from build123d import *

# Parameters (mm, degrees)
AUFSATZ_LINEAR_AUSTRAGEN1_DEPTH = 105
M5_GEWINDEBOHRUNG1_D            = 4.2
M5_GEWINDEBOHRUNG1_DEPTH        = 14
M5_GEWINDEBOHRUNG1_TIP          = 1.2618073
M5_GEWINDEBOHRUNG2_D            = 4.2
M5_GEWINDEBOHRUNG2_DEPTH        = 14
M5_GEWINDEBOHRUNG2_TIP          = 1.2618073
SKIZZE10_R                      = 2.55
SCHNITT_LINEAR_AUSTRAGEN1_DEPTH = 11
G1_4_GEWINDEBOHRUNG1_D          = 11.8


with BuildPart() as part:
    # Skizze1 → Aufsatz-Linear austragen1 (new body, symmetric)
    with BuildSketch(Plane.XY):
        Polygon((-40, 0), (40, 0), (40, 10), (10, 10), (10, 4), (-10, 4), (-10, 10), (-40, 10), align=None)
    extrude(amount=AUFSATZ_LINEAR_AUSTRAGEN1_DEPTH, both=True)

    # M5 Gewindebohrung1
    with Locations(Plane.XY.offset(105)):
        with Locations((-30, 4), (30, 4)):
            Hole(M5_GEWINDEBOHRUNG1_D / 2, depth=M5_GEWINDEBOHRUNG1_DEPTH)
            with Locations((0, 0, -(M5_GEWINDEBOHRUNG1_DEPTH + M5_GEWINDEBOHRUNG1_TIP / 2))):  # 118° drill point
                Cone(0, M5_GEWINDEBOHRUNG1_D / 2, M5_GEWINDEBOHRUNG1_TIP, mode=Mode.SUBTRACT)

    # M5 Gewindebohrung2
    with Locations(Plane(origin=(0, 0, -105), x_dir=(-1, 0, 0), z_dir=(0, 0, -1))):
        with Locations((-25, 4), (25, 4)):
            Hole(M5_GEWINDEBOHRUNG2_D / 2, depth=M5_GEWINDEBOHRUNG2_DEPTH)
            with Locations((0, 0, -(M5_GEWINDEBOHRUNG2_DEPTH + M5_GEWINDEBOHRUNG2_TIP / 2))):  # 118° drill point
                Cone(0, M5_GEWINDEBOHRUNG2_D / 2, M5_GEWINDEBOHRUNG2_TIP, mode=Mode.SUBTRACT)

    # Skizze10 → Schnitt-Linear austragen1 (cut, through all)
    with BuildSketch(Plane(origin=(0, 10, 0), x_dir=(1, 0, 0), z_dir=(0, 1, 0))):
        with Locations((25, 75)):
            Circle(SKIZZE10_R)
        with Locations((25, 45)):
            Circle(SKIZZE10_R)
        with Locations((25, 15)):
            Circle(SKIZZE10_R)
        with Locations((25, -15)):
            Circle(SKIZZE10_R)
        with Locations((25, -45)):
            Circle(SKIZZE10_R)
        with Locations((25, -75)):
            Circle(SKIZZE10_R)
        with Locations((-25, -75)):
            Circle(SKIZZE10_R)
        with Locations((-25, -45)):
            Circle(SKIZZE10_R)
        with Locations((-25, -15)):
            Circle(SKIZZE10_R)
        with Locations((-25, 15)):
            Circle(SKIZZE10_R)
        with Locations((-25, 45)):
            Circle(SKIZZE10_R)
        with Locations((-25, 75)):
            Circle(SKIZZE10_R)
    extrude(amount=-SCHNITT_LINEAR_AUSTRAGEN1_DEPTH, mode=Mode.SUBTRACT)

    # G1/4 Gewindebohrung1 (through all)
    with Locations(Plane(origin=(0, 4, 0), x_dir=(1, 0, 0), z_dir=(0, 1, 0))):
        with Locations((0, 95), (0, -95)):
            Hole(G1_4_GEWINDEBOHRUNG1_D / 2)


solid = part.part
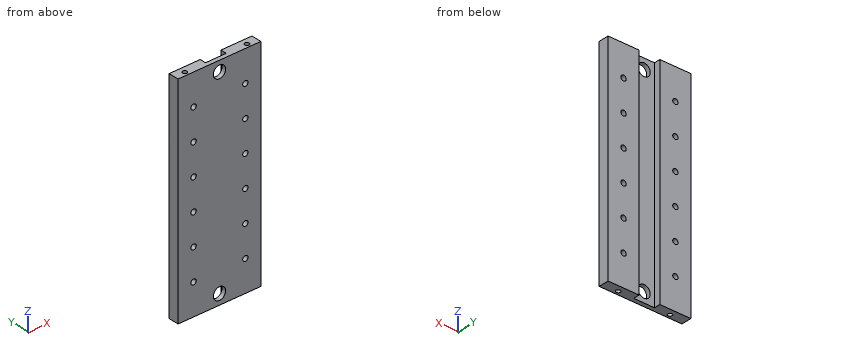
Can you work these out from the model? Positions are in its coordinate system, mm. Round coordinates to 2 decimals unless told otherwise and drop trailing zeros. Order: outer loops, then holes, each group sorted by start corner. A loop starts at its lowest first (then second) coordinate and runs counter-clockwise, first axis right, second up. Notation, with made-up numbers: M -32,87 L -26,87 A12 cw -26,106 Z; hole C -21.75,-10 d1. An arc over 180 degrees is marked long. Use a Markdown table: item, result.
1) I'm going to push flat-ended pins straight in: P1, Ø8, axis at x = -25, z = 15, coming from the +Y side; P2, Ø4, axis at x = 25, y = 4, coming from the -Z side. Where does each tip first touch, or does it pass through?
Geometry says:
| item | result |
|---|---|
| P1 | stops at y = 10 |
| P2 | stops at z = -90.94 |
2) If I drill on line 1 along X through (y, z) = (7.5, -15); line 2 along X through (y, z) = (8, 76.5); line 3 along X through (y, z) = (7.5, 94), over which ranges is the centre line in solid material (lowest first)?
Geometry says:
| item | result |
|---|---|
| line 1 | x = -40 to -27.55, -22.45 to -10, 10 to 22.45, 27.55 to 40 |
| line 2 | x = -40 to -27.06, -22.94 to -10, 10 to 22.94, 27.06 to 40 |
| line 3 | x = -40 to -10, 10 to 40 |
3) Imagine slicing it at D-D (z = -2). List the corners of the cut face in (x, y) for me, then the cut area to 3 significant figures.
Geometry says:
| item | result |
|---|---|
| outline | M -40,0 L 40,0 L 40,10 L 10,10 L 10,4 L -10,4 L -10,10 L -40,10 Z |
| area | 680 mm² |
4) Imagine slicing it at A-A (z = -95). List the corners of the cut face in (x, y) for me.
Geometry says:
| item | result |
|---|---|
| outline | M -40,0 L -5.9,0 L -5.9,4 L -10,4 L -10,10 L -40,10 Z; M 5.9,0 L 40,0 L 40,10 L 10,10 L 10,4 L 5.9,4 Z; hole C -25,4 d4.2; hole C 25,4 d4.2 |
5) Imagine slicing it at C-C (z = 75). List the corners of the cut face in (x, y) for me, then the cut area to 3 significant figures.
Geometry says:
| item | result |
|---|---|
| outline | M -40,0 L -27.55,0 L -27.55,10 L -40,10 Z; M -22.45,0 L 22.45,0 L 22.45,10 L 10,10 L 10,4 L -10,4 L -10,10 L -22.45,10 Z; M 27.55,0 L 40,0 L 40,10 L 27.55,10 Z |
| area | 578 mm² |
6) Imagine slicing it at B-B (x = 3). List the corners of the cut face in (y, z) for me, then the cut area to 3 significant figures.
Geometry says:
| item | result |
|---|---|
| outline | M 0,-105 L 4,-105 L 4,-100.08 L 0,-100.08 Z; M 0,-89.92 L 4,-89.92 L 4,89.92 L 0,89.92 Z; M 0,100.08 L 4,100.08 L 4,105 L 0,105 Z |
| area | 759 mm² |
